from build123d import *

# Parameters (mm, degrees)
SKETCH1_R           = 1.5
SKETCH1_R_2         = 32
BOSS_EXTRUDE1_DEPTH = 5
SKETCH1_31_R        = 12
BOSS_EXTRUDE2_DEPTH = 2
SKETCH1_32_W        = 6
SKETCH1_32_H        = 5
SKETCH1_32_R        = 0.5
BOSS_EXTRUDE3_DEPTH = 10
SKETCH1_33_W        = 37
SKETCH1_33_H        = 37
BOSS_EXTRUDE4_DEPTH = 17
SKETCH2_W           = 10
SKETCH2_H           = 4
CUT_EXTRUDE1_DEPTH  = 3.25


with BuildPart() as part:
    # Sketch1 → Boss-Extrude1 (new body)
    with BuildSketch(Plane.XY):
        with BuildLine():
            Line((-18.5, -41.733467654), (18.5, -41.733467654))
            Line((18.5, -41.733467654), (18.5, -35.464771253))
            ThreePointArc((18.5, -35.464771253), (0, 40), (-18.5, -35.464771253))
            Line((-18.5, -35.464771253), (-18.5, -41.733467654))
        make_face()
        with Locations((-20.57248383, -28.315594803)):
            Circle(SKETCH1_R, mode=Mode.SUBTRACT)
        with Locations((20.57248383, -28.315594803)):
            Circle(SKETCH1_R, mode=Mode.SUBTRACT)
        with Locations((-33.28697807, -10.815594803)):
            Circle(SKETCH1_R, mode=Mode.SUBTRACT)
        with Locations((-33.28697807, 10.815594803)):
            Circle(SKETCH1_R, mode=Mode.SUBTRACT)
        with Locations((-20.57248383, 28.315594803)):
            Circle(SKETCH1_R, mode=Mode.SUBTRACT)
        Circle(SKETCH1_R_2, mode=Mode.SUBTRACT)
        with Locations((33.28697807, -10.815594803)):
            Circle(SKETCH1_R, mode=Mode.SUBTRACT)
        with Locations((0, 35)):
            Circle(SKETCH1_R, mode=Mode.SUBTRACT)
        with Locations((33.28697807, 10.815594803)):
            Circle(SKETCH1_R, mode=Mode.SUBTRACT)
        with Locations((20.57248383, 28.315594803)):
            Circle(SKETCH1_R, mode=Mode.SUBTRACT)
    extrude(amount=BOSS_EXTRUDE1_DEPTH)



with BuildPart() as body_2:
    # Sketch1<31> → Boss-Extrude2 (new body)
    with BuildSketch(Plane.XY):
        Polygon((9.25, -49.983467654), (9.25, -44.983467654), (-9.25, -44.983467654), (-9.25, -49.983467654), (-15.25, -49.983467654), (-15.25, -70.483467654), (-9.25, -70.483467654), (-9.25, -75.483467654), (9.25, -75.483467654), (9.25, -70.483467654), (15.25, -70.483467654), (15.25, -49.983467654), align=None)
        with Locations((0, -60.233467654)):
            Circle(SKETCH1_31_R, mode=Mode.SUBTRACT)
    extrude(amount=BOSS_EXTRUDE2_DEPTH)

    # Sketch1<32> → Boss-Extrude3 (add)
    # profile 1 of 4: a face of its own
    with BuildSketch(Plane.XY):
        with Locations((-12.25, -47.483467654)):
            Rectangle(SKETCH1_32_W, SKETCH1_32_H)
        with Locations((-12.45, -48.456490694)):
            Circle(SKETCH1_32_R, mode=Mode.SUBTRACT)
    # profile 2 of 4: a face of its own
    with BuildSketch(Plane.XY):
        with Locations((12.25, -47.483467654)):
            Rectangle(SKETCH1_32_W, SKETCH1_32_H)
        with Locations((12.45, -48.456490694)):
            Circle(SKETCH1_32_R, mode=Mode.SUBTRACT)
    # profile 3 of 4: a face of its own
    with BuildSketch(Plane.XY):
        with Locations((12.25, -72.983467654)):
            Rectangle(SKETCH1_32_W, SKETCH1_32_H)
        with Locations((12.45, -72.010444613)):
            Circle(SKETCH1_32_R, mode=Mode.SUBTRACT)
    # profile 4 of 4: a face of its own
    with BuildSketch(Plane.XY):
        with Locations((-12.25, -72.983467654)):
            Rectangle(SKETCH1_32_W, SKETCH1_32_H)
        with Locations((-12.45, -72.010444613)):
            Circle(SKETCH1_32_R, mode=Mode.SUBTRACT)
    extrude(amount=BOSS_EXTRUDE3_DEPTH)


with BuildPart() as part_1:
    add(part.part)

    add(body_2.part)  # Boss-Extrude4 merges body 2
    # Sketch1<33> → Boss-Extrude4 (add)
    with BuildSketch(Plane.XY):
        with Locations((0, -60.233467654)):
            Rectangle(SKETCH1_33_W, SKETCH1_33_H)
        Polygon((9.25, -44.983467654), (15.25, -44.983467654), (15.25, -49.983467654), (15.25, -70.483467654), (15.25, -75.483467654), (9.25, -75.483467654), (-9.25, -75.483467654), (-15.25, -75.483467654), (-15.25, -70.483467654), (-15.25, -49.983467654), (-15.25, -44.983467654), (-9.25, -44.983467654), align=None, mode=Mode.SUBTRACT)
    extrude(amount=BOSS_EXTRUDE4_DEPTH)

    # Sketch2 → Cut-Extrude1 (cut)
    with BuildSketch(Plane.XZ.offset(44.983467654)):
        with Locations((0, 15)):
            Rectangle(SKETCH2_W, SKETCH2_H)
    extrude(amount=-CUT_EXTRUDE1_DEPTH, mode=Mode.SUBTRACT)


solid = part_1.part
Can you work these out from the model? Positions are in its coordinate system, mm. A direction names the side the tool comes from. Round coordinates to 2 decimals unless told otherwise and drop trailing zeros. Write each loop counter-clockwise with the first axis right and the second up, starting at its lowest first coordinate (ties: lowest second). Pieces come first, ordered by that corner, then holes. Notation, with made-up numbers: (83, 16.5) -> (99, 16.5) arc R27 cw to (99, 37.5) -> close; hole circle Ø10 at (-18, 53.25). An arc over 180 degrees is marked (long way). One line per question, with ' | ' between items. Start each with the question number.
1) Suppose I cut it at B-B on x = 30. Write out the boundary of the cut face in (y, z), then the cut area to 3 significant figures.
2) On a 3-axis mill with a long thin cutter (end or side, diameter ignored), from which of +Z, -Z, +X, -X, +Y, -Y can I reach the whole of each face in a straight line? I mean faces 1 (the flat face through (-12, -47, 10)), 2 (the flat face through (0, -77, 17)), 3 (the flat face through (0, -41.733, 11)). Say none if no direction works.
3) Suppose I cut it at C-C on z = 3.25. Count the separate pieces of the cut face and the enclosed holes in it, then the cut area to 3 significant figures.
4) If we mould it in two halves opening along X, with no side actions, what happens to faces 4 (the flat face through (-18.5, -57, 8)), 5 (the cylindrical face through (-1.562, -48.336, 0.986)), 6 (the flat face through (0, -78.733, 8))? For each: released by +X, released by -X, zero draft, split by the parting line, or undercut.
5) Suppose I cut it at A-A on y = 0. Write out the boundary of the cut face in (x, z), then the cut area to 3 significant figures.
6) I need wall thicknesses on line 1 (Y direction, x = 0, z = 1.4); line 2 (Y direction, x = -12.45, z = 6.5); line 3 (Y direction, x = 7, z = 5.25). Which ranges of each line are inside material? Lowest first, please. Write a range as [from, to].
7) I'm going to push flat-ended pins straight in: P1, Ø3, axis at x = 11.5, z = 7.5, coming from the +Y side; P2, Ø2.5, axis at x = -12.5, y = -74, coming from the +Z side; P3, Ø5.5, axis at y = -47.5, z = 5, coming from the -X side. Where does each tip first touch, or does it pass through?
8) Suppose I cut it at D-D on z = 15.75. Write out the boundary of the cut face in (x, y), then the cut area to 3 significant figures.
Return value:
1) outline: (-26.46, 0) -> (-11.14, 0) -> (-11.14, 5) -> (-26.46, 5) -> close; (11.14, 0) -> (26.46, 0) -> (26.46, 5) -> (11.14, 5) -> close | area: 153 mm2
2) face 1: +Z | face 2: +Z, +X, -X, +Y, -Y | face 3: +Z, +X, -X, +Y
3) separate pieces: 1 | enclosed holes: 15 | area: 2,420 mm2
4) face 4: released by -X | face 5: undercut | face 6: zero draft
5) outline: (-40, 0) -> (-32, 0) -> (-32, 5) -> (-40, 5) -> close; (32, 0) -> (40, 0) -> (40, 5) -> (32, 5) -> close | area: 80.0 mm2
6) line 1: y = [-78.73, -72.23], [-48.23, -32], [32, 33.5], [36.5, 40] | line 2: y = [-78.73, -72.51], [-71.51, -70.48], [-49.98, -48.96], [-47.96, -41.73] | line 3: y = [-78.73, -75.48], [-44.98, -41.73]
7) P1: stops at y = -41.73 | P2: stops at z = 10 | P3: stops at x = -18.5
8) outline: (-18.5, -78.73) -> (18.5, -78.73) -> (18.5, -41.73) -> (5, -41.73) -> (5, -44.98) -> (15.25, -44.98) -> (15.25, -75.48) -> (-15.25, -75.48) -> (-15.25, -44.98) -> (-5, -44.98) -> (-5, -41.73) -> (-18.5, -41.73) -> close | area: 406 mm2
